```python
from build123d import *

# Parameters (mm, degrees)
SKETCH2_W               = 444.5
SKETCH2_H               = 584.2
BOSS_EXTRUDE1_DEPTH     = 6.35
MOVE_START              = -2.17182791
MOVE_FACE1_OUTLINE_W    = 448
MOVE_FACE1_OUTLINE_H    = 9
MOVE_FACE1_DEPTH        = 2.17182791
CONVERT_SOLID1_START    = -222.25
CONVERT_SOLID1_DEPTH    = 444.5
SKETCH7_W               = 19.05
SKETCH7_H               = 5.08
CUT_EXTRUDE1_DEPTH      = 626.080014878
SKETCH9_R               = 1.905
CUT_EXTRUDE2_DEPTH      = 1.2192
CHAMFER1_SIZE           = 2.54
CUT_EXTRUDE3_DEPTH      = 626.080014878
CUT_EXTRUDE3_DEPTH_BACK = 626.080014878
SKETCH10_R              = 12.7


# Read off the part's stored shape, not the designer's step: Move Face1, Convert-Solid1
with BuildPart() as part:
    # Sketch2 → Boss-Extrude1 (new body)
    with BuildSketch(Plane(origin=(0, 0, 0), x_dir=(1, 0, 0), z_dir=(0, 1, 0))):
        with Locations((0, 292.1)):
            Rectangle(SKETCH2_W, SKETCH2_H)
    extrude(amount=-BOSS_EXTRUDE1_DEPTH)

    # Move Face1 outline → Move Face1 (cut)
    with BuildSketch(Plane(origin=(0, 0, 0), x_dir=(1, 0, 0), z_dir=(0, 0.3420201433256691, -0.9396926207859083)).offset(MOVE_START)):
        with Locations((0, 3.5)):
            Rectangle(MOVE_FACE1_OUTLINE_W, MOVE_FACE1_OUTLINE_H)
    extrude(amount=MOVE_FACE1_DEPTH, mode=Mode.SUBTRACT)

    # Convert-Solid1 outline → Convert-Solid1 (cut)
    with BuildSketch(Plane.YZ.offset(CONVERT_SOLID1_START)):
        with BuildLine():
            Line((-6.037256781, -3.17046592), (-6.35, -2.311210988))
            Line((-6.35, -2.311210988), (-6.35, -583.2856))
            Line((-6.35, -583.2856), (-1.6764, -583.2856))
            ThreePointArc((-1.6764, -583.2856), (-1.137584633, -583.062415367), (-0.9144, -582.5236))
            Line((-0.9144, -582.5236), (-0.9144, -2.394147319))
            ThreePointArc((-0.9144, -2.394147319), (-1.239334756, -1.769953461), (-1.937019349, -1.678101541))
            Line((-1.937019349, -1.678101541), (-6.037256781, -3.17046592))
        make_face()
        with BuildLine():
            Line((0, 0), (-2.249762568, -0.818846609))
            ThreePointArc((-2.249762568, -0.818846609), (-0.714856462, -1.020920831), (0, -2.394147319))
            Line((0, -2.394147319), (0, 0))
        make_face()
        with BuildLine():
            Line((0, -584.2), (0, -582.5236))
            ThreePointArc((0, -582.5236), (-0.491006192, -583.708993808), (-1.6764, -584.2))
            Line((-1.6764, -584.2), (0, -584.2))
        make_face()
    extrude(amount=CONVERT_SOLID1_DEPTH, mode=Mode.SUBTRACT)

    # Sketch7 → Cut-Extrude1 (cut, through all)
    with BuildSketch(Plane(origin=(0, 0, 0), x_dir=(1, 0, 0), z_dir=(0, 1, 0))):
        with Locations((-212.725, 2.54)):
            Rectangle(SKETCH7_W, SKETCH7_H)
        with Locations((212.725, 2.54)):
            Rectangle(SKETCH7_W, SKETCH7_H)
    extrude(amount=-CUT_EXTRUDE1_DEPTH, mode=Mode.SUBTRACT)

    # Sketch9 → Cut-Extrude2 (cut)
    with BuildSketch(Plane(origin=(0, 0, 0), x_dir=(1, 0, 0), z_dir=(0, 1, 0))):
        with Locations(Location((-210.82, 25.4, 0), (0, 0, 270))):
            Circle(SKETCH9_R)
        with Locations(Location((-210.82, 317.5, 0), (0, 0, 270))):
            Circle(SKETCH9_R)
        with Locations(Location((-210.82, 558.8, 0), (0, 0, 270))):
            Circle(SKETCH9_R)
        with Locations(Location((210.82, 558.8, 0), (0, 0, 90))):
            Circle(SKETCH9_R)
        with Locations(Location((210.82, 317.5, 0), (0, 0, 90))):
            Circle(SKETCH9_R)
        with Locations(Location((210.82, 25.4, 0), (0, 0, 90))):
            Circle(SKETCH9_R)
        with BuildLine():
            Line((-43.0182, 465.455), (-45.0182, 465.455))
            ThreePointArc((-45.0182, 465.455), (-46.9232, 467.36), (-45.0182, 469.265))
            Line((-45.0182, 469.265), (-43.0182, 469.265))
            ThreePointArc((-43.0182, 469.265), (-41.1132, 467.36), (-43.0182, 465.455))
        make_face()
        with BuildLine():
            Line((45.0182, 465.455), (43.0182, 465.455))
            ThreePointArc((43.0182, 465.455), (41.1132, 467.36), (43.0182, 469.265))
            Line((43.0182, 469.265), (45.0182, 469.265))
            ThreePointArc((45.0182, 469.265), (46.9232, 467.36), (45.0182, 465.455))
        make_face()
        with BuildLine():
            Line((-43.0182, 165.735), (-45.0182, 165.735))
            ThreePointArc((-45.0182, 165.735), (-46.9232, 167.64), (-45.0182, 169.545))
            Line((-45.0182, 169.545), (-43.0182, 169.545))
            ThreePointArc((-43.0182, 169.545), (-41.1132, 167.64), (-43.0182, 165.735))
        make_face()
        with BuildLine():
            Line((45.0182, 165.735), (43.0182, 165.735))
            ThreePointArc((43.0182, 165.735), (41.1132, 167.64), (43.0182, 169.545))
            Line((43.0182, 169.545), (45.0182, 169.545))
            ThreePointArc((45.0182, 169.545), (46.9232, 167.64), (45.0182, 165.735))
        make_face()
    extrude(amount=-CUT_EXTRUDE2_DEPTH, mode=Mode.SUBTRACT)

    # Chamfer1
    chamfer1_edges = [part.edges().sort_by_distance(p)[0] for p in [
        (-222.25, -6.35, -583.7428),
        (222.25, -6.35, -583.7428),
        (-222.25, -0.4572, -5.08),
        (-203.2, -6.193628391, -2.740838454),
        (222.25, -0.4572, -5.08),
        (203.2, -6.193628391, -2.740838454),
    ]]
    chamfer(chamfer1_edges, length=CHAMFER1_SIZE)

    # Sketch10 → Cut-Extrude3 (cut, two sides: drawn at the far end of the back side and taken through both)
    with BuildSketch(Plane(origin=(0, 0, 0), x_dir=(1, 0, 0), z_dir=(0, 1, 0)).offset(-CUT_EXTRUDE3_DEPTH_BACK)):
        with Locations(Location((18.542, 162.007747319, 0), (0, 0, 270))):
            Circle(SKETCH10_R)
        with Locations(Location((-16.51, 17.78, 0), (0, 0, 270))):
            Circle(SKETCH10_R)
        with Locations(Location((-31.75, 246.38, 0), (0, 0, 270))):
            Circle(SKETCH10_R)
        with Locations(Location((118.11, 17.78, 0), (0, 0, 270))):
            Circle(SKETCH10_R)
        with Locations(Location((-27.94, 513.08, 0), (0, 0, 270))):
            Circle(SKETCH10_R)
        with Locations(Location((27.94, 121.92, 0), (0, 0, 270))):
            Circle(SKETCH10_R)
    extrude(amount=CUT_EXTRUDE3_DEPTH + CUT_EXTRUDE3_DEPTH_BACK, mode=Mode.SUBTRACT)


solid = part.part
```
Can you work these out from the model? Positions are in its coordinate system, mm. Coordinates: 2 decimals unless noted, no trailing zeros. Loops run counter-clockwise (first coordinate to the right, second up) from the corner with the lowest first, then second, coordinate; pieces in that order, holes last.
Item 1: Suppose I cut it at C-C (z = -305). Please give me the cut outline in (x, y), then the cut area to 3 significant figures.
Answers below:
outline: (-222.25, -0.91) - (222.25, -0.91) - (222.25, 0) - (-222.25, 0) - close
area: 406 mm2
Item 2: Please list where these lines run through material, in increasing order: L1, parallel to X at y = -0.3, z = -317.5 (3 decimals); L2, parallel to Z at x = -134.5, y = -2; L3, parallel to Z at x = 210.82, y = -0.45 (3 decimals).
Answers below:
L1: x = -222.25 to -212.725, -208.915 to 208.915, 212.725 to 222.25
L2: z = -584.2 to -583.29, -1.7 to -0.75
L3: z = -583.667 to -560.705, -556.895 to -319.405, -315.595 to -27.305, -23.495 to -5.08
Item 3: If we mould it in two halves opening along Z, with no side actions, what happens to faces 1 (the face through (130.702, -0.464, -19.433)), 2 (the face through (-3, 0, -297))? For each: released by +Z, released by -Z, zero draft, split by the parting line, or undercut.
Answers below:
face 1: undercut
face 2: zero draft
Item 4: Suppose I cut it at B-B (x = -153). Please give me the cut outline in (y, z), then the cut area to 3 significant figures.
Answers below:
outline: (-6.35, -584.2) - (-1.68, -584.2) arc R1.68 ccw to (0, -582.52) - (0, -2.39) arc R1.68 ccw to (-2.25, -0.82) - (-6.35, -2.31) - (-6.04, -3.17) - (-1.94, -1.68) arc R0.76 cw to (-0.91, -2.39) - (-0.91, -582.52) arc R0.76 cw to (-1.68, -583.29) - (-6.35, -583.29) - close
area: 543 mm2
Item 5: Suppose I cut it at A-A (z = -121.92). Please give me the cut outline in (x, y), then the cut area to 3 significant figures.
Answers below:
outline: (-222.25, -0.91) - (15.24, -0.91) - (15.24, 0) - (-222.25, 0) - close; (40.64, -0.91) - (222.25, -0.91) - (222.25, 0) - (40.64, 0) - close
area: 383 mm2
Item 6: I'm going to push flat-ended pins straight in: pin 1 (4 mm diameter, centred on x = 37, z = -206, fed in from -Y); pin 2 (2 mm diameter, centred on y = -2, z = -4, fed in from -X); pin 3 (0.5 mm diameter, centred on x = -44, y = -0.5, fed in from +Z); pin 4 (0.7 mm diameter, centred on x = -44, y = -0.5, fed in from -Z). Where does each tip first touch, or does it pass through?
Answers below:
pin 1: stops at y = -0.91
pin 2: passes through
pin 3: stops at z = -1
pin 4: stops at z = -583.98
